Here's how the part is built. I have some questions about the finished solid (model axes, mm). Face numbers are marked on the shaded views. A direction names the side the tool comes from. Give positions to 0.01 mm unless a question says otherwise; leave off trailing zeros. Loops run counter-clockwise (first coordinate to the right, second up) from the corner with the lowest first, then second, coordinate; pieces in that order, holes last. Notation, with made-up numbers: M -4,53 L 52,53 A13 cw 52,78 Z; hole C 84.25,-31.75 d1. An arc over 180 degrees is marked long. Write item = value, one per line. Start each with the question number.
Autodesk Inventor part; units mm, degrees
ref_plane "YZ Plane" through (0, 0, 0) normal (1, 0, 0) x (0, 1, 0)
ref_plane "XZ Plane" through (0, 0, 0) normal (0, 1, 0) x (-1, 0, 0)
ref_plane "XY Plane" through (0, 0, 0) normal (0, 0, 1) x (1, 0, 0)
sketch "Sketch1" plane through (0, 0, 0) normal (0, 1, 0) x (-1, 0, 0)
  line L0 (-90, 35) -> (90, 35)
  line L1 (90, 35) -> (90, -35)
  line L2 (90, -35) -> (-90, -35)
  line L3 (-90, -35) -> (-90, 35)
  line L4 (-90, 35) -> (90, -35) construction
  line L5 (90, 35) -> (-90, -35) construction
  point P0 (0, 0)
  dimension "d0" = 70
  dimension "d1" = 180
extrude "Plate1" add sketch "Sketch1" along normal blind 3
sketch "Sketch2" plane through (87.0114, 3.2615, 35) normal (0.9961947, -0.0871557, 0) x (0.0871557, 0.9961947, 0)
  line L0 (0, -70) -> (0, 0)
  line L1 (0, 0) -> (-50, 0)
  line L2 (-50, 0) -> (-50, -70)
  line L3 (-50, -70) -> (0, -70)
edge flange "Flange1" height 50 angle 95 thickness 3 bend radius 3 thickness toward (0.9961947, -0.0871557, 0) relief tear relief width 3 relief depth 1.5 edges at (90, 0, 0) wall of the first edge with corners at (87.0114, 3.2615, -35) (87.0114, 3.2615, 35) (82.6536, -46.5483, 35) (82.6536, -46.5483, -35)
bend "Bend1"
corner "Corner1"
sketch "Sketch3" plane through (0, 3, 0) normal (0, 1, 0) x (1, 0, 0)
  line L0 (-43.6, -26.2) -> (-80, -26.2) construction
  line L1 (-80, -26.2) -> (-80, 26.2) construction
  line L2 (-80, 26.2) -> (-43.6, 26.2) construction
  line L3 (-43.6, 26.2) -> (-43.6, -26.2) construction
  line L4 (-43.6, -26.2) -> (-80, 26.2) construction
  line L5 (-80, -26.2) -> (-43.6, 26.2) construction
  line L6 (-90, -35) -> (-90, 35) construction
  point P0 (0, 0)
  point P1 (-61.8, 0)
  dimension "d13" = 52.4
  dimension "d14" = 36.4
  dimension "d15" = 10
hole "Hole1" at (-80, 3, 26.2) at (-80, 3, -26.2) at (-43.6, 3, -26.2) at (-43.6, 3, 26.2) direction (0, -1, 0) diameter 4.8 end through all
sketch "Sketch4" plane through (82.6536, -46.5483, -35) normal (-0.9961947, 0.0871557, 0) x (0, 0, 1)
  line L0 (12.5, 13.5) -> (57.5, 13.5) construction
  line L1 (57.5, 13.5) -> (57.5, 29.9521) construction
  line L2 (57.5, 29.9521) -> (12.5, 29.9521) construction
  line L3 (12.5, 29.9521) -> (12.5, 13.5) construction
  line L4 (12.5, 13.5) -> (57.5, 29.9521) construction
  line L5 (57.5, 13.5) -> (12.5, 29.9521) construction
  line L6 (70, 43.4521) -> (0, 43.4521) construction
  line L7 (0, 43.4521) -> (0, 0) construction
  line L8 (0, 0) -> (70, 0) construction
  line L9 (70, 43.4521) -> (70, 0) construction
  circle A0 centre (57.5, 29.9521) radius 2.75
  line L10 (53.5346, 32.7021) -> (62.0591, 32.7021)
  point P0 (35, 39.1674)
  point P1 (35, 21.7261)
  point P2 (70, 21.7261)
  dimension "d23" = 0
  dimension "d24" = 70
  dimension "d25" = 45
  dimension "d26" = 13.5
  dimension "d27" = 16.4521
  dimension "d28" = 5.5
  dimension "d29" = 10.75
hole "Hole2" at (85.2641, -16.7101, -22.5) at (83.8302, -33.0996, -22.5) at (85.2641, -16.7101, 22.5) at (83.8302, -33.0996, 22.5) direction (0.9961947, -0.0871557, 0) diameter 5.5 end through all
fillet "Fillet1" radius 5 4 edges at (84.1479, -46.679, 35) (84.1479, -46.679, -35) (-90, 1.5, 35) (-90, 1.5, -35)
equation "\"d21\" = Thickness"
equation "\"d35\" = Thickness"
equation "\"d2\" = Thickness"
equation "\"d3\" = BendReliefWidth"
equation "\"d4\" = BendReliefDepth"
equation "\"d5\" = MinimumRemnant"
equation "\"d6\" = TransitionRadius"
equation "\"d9\" = BendRadius"
equation "\"d10\" = CornerReliefSize"
equation "\"d11\" = GapSize"
equation "\"d12\" = JacobiRadiusSize"
equation "\"BendRadius\" = Thickness"
equation "\"BendReliefWidth\" = Thickness"
equation "\"BendReliefDepth\" = 0.5 * Thickness"
equation "\"CornerReliefSize\" = 4 * Thickness"
equation "\"MinimumRemnant\" = 2 * Thickness"
equation "\"TransitionRadius\" = BendRadius"
equation "\"JacobiRadiusSize\" = BendRadius"
equation "\"GapSize\" = Thickness"
properties part number "26062025_2" material "AISI 304"
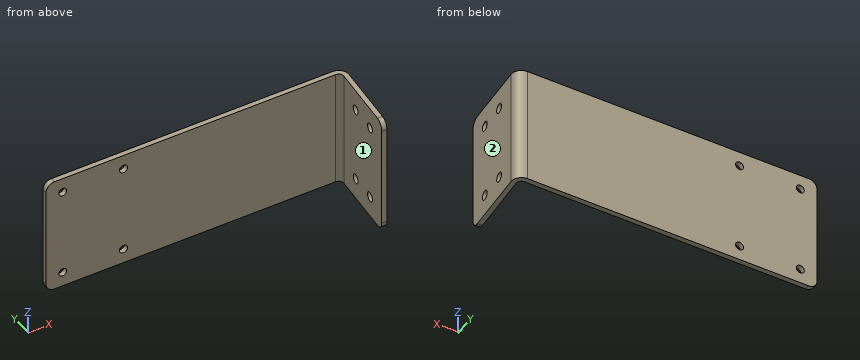
Q1. If I drill on line 1 along Z through (x, y) = (-43.6, 1.45); line 2 along X through (y, z) = (1.8, -26.2); line 3 along X through (y, z) = (2.1, 26.2), over which ranges is the centre line in solid material (lowest first)?
Q2. If we section it at C-C, the plane x = 36: List the corners of the cut face in (y, z) for me, then the cut area to 3 significant figures.
Q3. On a 3-axis mill with a long thin cutter (end or side, diameter ignored), from which of +Z, -Z, +X, -X, +Y, -Y can I reach the whole of each face in a straight line? I mean the marked faces 1 and 2. Say none if no direction works.
Q4. Will these pins go through, and if not, where does the flat tip stop? pin 1 (1.5 mm diameter, centred on y = -32, z = -13, fed in from -X); pin 2 (8 mm diameter, centred on y = -37.5, z = -14, fed in from -X); pin 3 (6 mm diameter, centred on y = -6, z = -26.5, fed in from +X); pin 4 (1.5 mm diameter, centred on x = 27.5, z = -8, fed in from -Y).
Q5. If we section it at A-A, the plane x = -43.6: List the corners of the cut face in (y, z) for me, then the cut area to 3 significant figures.
Q6. If we section it at B-B, the plane z = -21.5: List the corners of the cut face in (x, y) for me.
Resolved:
q1.line_1 = -35 to -28.6, -23.8 to 23.8, 28.6 to 35
q1.line_2 = -90 to -82.4, -77.6 to -46, -41.2 to 87.05
q1.line_3 = -90 to -82.4, -77.6 to -46, -41.2 to 86.61
q2.outline = M 0,-35 L 3,-35 L 3,35 L 0,35 Z
q2.area = 210 mm²
q3.face_1 = +Z, -Z, -X
q3.face_2 = +Z, -Z, +X, -Y
q4.pin_1 = 83.86
q4.pin_2 = 83.1
q4.pin_3 = 89.45
q4.pin_4 = 0
q5.outline = M 0,-35 L 3,-35 L 3,-28.6 L 0,-28.6 Z; M 0,-23.8 L 3,-23.8 L 3,23.8 L 0,23.8 Z; M 0,28.6 L 3,28.6 L 3,35 L 0,35 Z
q5.area = 181 mm²
q6.outline = M -90,0 L 83.45,0 A3 cw 86.44,-3.26 L 85.49,-14.16 L 88.48,-14.42 L 89.43,-3.52 A6 ccw 83.45,3 L -90,3 Z; M 82.65,-46.55 L 85.64,-46.81 L 86.6,-35.91 L 83.61,-35.65 Z; M 84.05,-30.55 L 87.04,-30.81 L 88.03,-19.52 L 85.04,-19.26 Z
